Source: CAD feature listing. Evaluate the final solid. Frame: model axes, mm. A direction names the side the tool comes from. Round coordinates to 2 decimals unless told otherwise and drop trailing zeros. Loops run counter-clockwise (first coordinate to the right, second up) from the corner with the lowest first, then second, coordinate; pieces in that order, holes last. Notation, with made-up numbers: (66.5, 34) - (105.5, 34) arc R25 cw to (105.5, 50) - close; hole circle Ø10 at (-17, 60). An arc over 180 degrees is marked (long way). One line per question, with ' | ' between items. Start each with the question number.
1. Cut plane A-A (y = 6.2). Return loops of the section in (x, z).
2. Pin query (flat end, axial travel): pin 1 (5 mm diameter, centred on y = 31, z = 16, fed in from -X); pin 2 (14.5 mm diameter, centred on y = 6.5, z = 22.5, fed in from -X); pin 3 (15.5 mm diameter, centred on x = -24, z = 25, fed in from -Y). Return the tip coordinate at first contact, or that it passes through.
3. Ray query, line 1 (Y direction, x = -7.9, z = 15); line 2 (Z direction, x = -7, y = 6); line 3 (Y direction, x = -45.5, z = 17.5). Return the intervals inside material, ascending.
4. Cut plane D-D (x = -17.5). Return loops of the section in (y, z), then the cut area to 3 significant figures.
5. Access query for faces 1 (the flat face through (-48, 49, 30)), 2 (the flat face through (-49, 43, 30)), 3 (the flat face through (-6, 8, 30)). Directions: +Z, -Z, +X, -X, +Y, -Y. A direction counts if a zero-diameter tool reaches every point of the face in a straight line with its end or side. Return the directions, or none.
6. Cut plane B-B (z = 52). State how many separate pieces and enclosed holes the cut face has, then the cut area to 3 significant figures.
7. Mould query, pull axis X, two halves, no side actions, for faces 4 (the flat face through (-40.2, 47, 30)), 5 (the flat face through (-3, 7, 30)), 6 (the flat face through (-43, 52, 30)). Classes: pulls with the +X half, pulls with the -X half, needs draft (parallel to the pull), parting line crosses it, or undercut.
8. Cut plane C-C (z = 28.5). Return loops of the section in (x, y), then the cut area to 3 significant figures.
```python
from build123d import *

# Parameters (mm, degrees)
DODANIE_WYCI_GNI_CIE1_DEPTH = 60
SFAZOWANIE1_SIZE            = 2
SZKIC2_R                    = 3.1
WYTNIJ_WYCI_GNI_CIE1_DEPTH  = 10
SZKIC3_R                    = 2.1
WYTNIJ_WYCI_GNI_CIE2_DEPTH  = 10
SZKIC4_R                    = 2.1
WYTNIJ_WYCI_GNI_CIE3_DEPTH  = 10


with BuildPart() as part:
    # Szkic1 → Dodanie-wyciągnięcie1 (new body)
    with BuildSketch(Plane.XY):
        Polygon((0, 0), (-3, 0), (-3, 15), (-6, 15), (-6, 0), (-9, 0), (-9, 15), (-30.2, 15), (-40.2, 25), (-40.2, 43), (-55.2, 43), (-55.2, 46), (-40.2, 46), (-40.2, 49), (-55.2, 49), (-55.2, 52), (-30.2, 52), (-30.2, 25), (0, 25), align=None)
    extrude(amount=DODANIE_WYCI_GNI_CIE1_DEPTH)

    # Sfazowanie1
    sfazowanie1_edges = [part.edges().sort_by_distance(p)[0] for p in [
        (-9, 15, 30),
        (-40.2, 43, 30),
    ]]
    chamfer(sfazowanie1_edges, length=SFAZOWANIE1_SIZE)

    # Szkic2 → Wytnij-wyciągnięcie1 (cut)
    with BuildSketch(Plane.XZ.offset(-43)):
        with Locations(Location((-48.5, 52, 0), (0, 0, 270))):
            Circle(SZKIC2_R)
    extrude(amount=-WYTNIJ_WYCI_GNI_CIE1_DEPTH, mode=Mode.SUBTRACT)

    # Szkic3 → Wytnij-wyciągnięcie2 (cut)
    with BuildSketch(Plane.XZ.offset(-43)):
        with Locations(Location((-49.2, 15, 0), (0, 0, 270))):
            Circle(SZKIC3_R)
    extrude(amount=-WYTNIJ_WYCI_GNI_CIE2_DEPTH, mode=Mode.SUBTRACT)

    # Szkic4 → Wytnij-wyciągnięcie3 (cut)
    with BuildSketch(Plane.ZY.offset(9)):
        with Locations((15, 6.2)):
            Circle(SZKIC4_R)
    extrude(amount=-WYTNIJ_WYCI_GNI_CIE3_DEPTH, mode=Mode.SUBTRACT)


solid = part.part
```
Answers follow:
1) outline: (-9, 0) - (-6, 0) - (-6, 12.9) - (-9, 12.9) - close; (-9, 17.1) - (-6, 17.1) - (-6, 60) - (-9, 60) - close; (-3, 0) - (0, 0) - (0, 12.9) - (-3, 12.9) - close; (-3, 17.1) - (0, 17.1) - (0, 60) - (-3, 60) - close
2) pin 1: stops at x = -40.2 | pin 2: stops at x = -9.75 | pin 3: stops at y = 15
3) line 1: y = 0 to 4.1, 8.3 to 25 | line 2: z = 0 to 12.91, 17.09 to 60 | line 3: y = 43 to 46, 49 to 52
4) outline: (15, 0) - (25, 0) - (25, 60) - (15, 60) - close | area: 600 mm2
5) face 1: +Z, -Z, -X | face 2: +Z, -Z, -X, -Y | face 3: +Z, -Z, -Y
6) separate pieces: 3 | enclosed holes: 0 | area: 769 mm2
7) face 4: pulls with the -X half | face 5: undercut | face 6: needs draft
8) outline: (-55.2, 43) - (-42.2, 43) - (-40.2, 41) - (-40.2, 25) - (-30.2, 15) - (-11, 15) - (-9, 13) - (-9, 0) - (-6, 0) - (-6, 15) - (-3, 15) - (-3, 0) - (0, 0) - (0, 25) - (-30.2, 25) - (-30.2, 52) - (-55.2, 52) - (-55.2, 49) - (-40.2, 49) - (-40.2, 46) - (-55.2, 46) - close | area: 806 mm2
